Source: CAD feature listing. Evaluate the final solid. Frame: model axes, mm. A direction names the side the tool comes from. Give positions to 0.01 mm unless a question says otherwise; leave off trailing zeros. Loops run counter-clockwise (first coordinate to the right, second up) from the corner with the lowest first, then second, coordinate; pieces in that order, holes last. Notation, with made-up numbers: M -25,-6.5 L 17,-6.5 A34 ccw 17,32.5 Z; hole C 25,76 d10. An arc over 180 degrees is marked long. Put each result on its own line as item: value. Start each with the question number.
```python
from build123d import *

# Parameters (mm, degrees)
F0_R     = 1.539144
F0_R_2   = 1.452362
F0_R_3   = 1.631379
F0_R_4   = 1.528566
F0_R_5   = 1.549722
F0_R_6   = 5.024672
F0_R_7   = 1.528565
F1_DEPTH = 4


with BuildPart() as f1:
    # F0 (on Top) → F1 (new body)
    with BuildSketch(Plane.XY):
        Polygon((18.500502, 18), (-35.499498, 18), (-35.499498, 0), (18.500502, 0), (30.500502, -7), (42.500502, -7), (54.500502, 0), (54.500502, 18), (42.500502, 25), (30.500502, 25), align=None)
        with Locations((-28.499498, 3.5)):
            Circle(F0_R, mode=Mode.SUBTRACT)
        with Locations((29.135042, 3)):
            Circle(F0_R_2, mode=Mode.SUBTRACT)
        with Locations((41.504552, 2.758247)):
            Circle(F0_R_3, mode=Mode.SUBTRACT)
        with Locations((-28.499498, 14.5)):
            Circle(F0_R_4, mode=Mode.SUBTRACT)
        with Locations((31.46798, 15.21882)):
            Circle(F0_R_5, mode=Mode.SUBTRACT)
        with Locations((36.500502, 9)):
            Circle(F0_R_6, mode=Mode.SUBTRACT)
        with Locations((43.865962, 15)):
            Circle(F0_R_7, mode=Mode.SUBTRACT)
    extrude(amount=F1_DEPTH)


solid = f1.part
```
1. Section A-A, the plane y = 9. Output: boundary loops of the cut face in (x, z), plus the area to 3 significant figures.
2. Pull-direction query (X, two-part tool) for faces 4 (the face through (37, 25, 2)), 5 (the face through (54.501, 9, 2)), 6 (the face through (39.875, 2.83, 1.972)); classes: released by +X, released by -X, zero draft, split by the parting line, or undercut.
3. Section C-C, the plane x = 8. Output: boundary loops of the cut face in (y, z), plus the area to 3 significant figures.
4. Section D-D, the plane y = 19.5. Output: boundary loops of the cut face in (x, z).
5. Ray query, line 1 (Y direction, x = 8.5, z = 3.8); line 2 (X direction, y = 5.5, z = 0.3); line 3 (Y direction, x = 34, z = 3.6). Return the intervals inside material, ascending.
6. Set-up query: faces 1 (the face through (-9, 0, 2)), 2 (the face through (36, -7, 2)), 3 (the face through (-8, 18, 2)). Return all of +Z, -Z, +X, -X, +Y, -Y with unobstructed straight access to the full face (end or side cutting, diameter ignored); none if empty.
7. Contact query for flat-ended pins moving along their axis: pin 1 (1.9 mm diameter, centred on x = 31.47, y = 15.22, fed in from -Z); pin 2 (1 mm diameter, centred on x = 44.5, z = 1.5, fed in from -Y); pin 3 (1.2 mm diameter, centred on x = -21, z = 1.5, fed in from -Y). Output: stop coordinate, or through.
8. Section B-B, the plane z = 2.5. Output: boundary loops of the cut face in (x, y).
Results found:
1. outline: M -35.5,0 L 31.48,0 L 31.48,4 L -35.5,4 Z; M 41.53,0 L 54.5,0 L 54.5,4 L 41.53,4 Z
1. area: 320 mm²
2. face 4: zero draft
2. face 5: released by +X
2. face 6: undercut
3. outline: M 0,0 L 18,0 L 18,4 L 0,4 Z
3. area: 72.0 mm²
4. outline: M 21.07,0 L 51.93,0 L 51.93,4 L 21.07,4 Z
5. line 1: 0 to 18
5. line 2: -35.5 to 32.9, 40.11 to 54.5
5. line 3: -7 to 4.64, 13.36 to 25
6. face 1: +Z, -Z, -X, -Y
6. face 2: +Z, -Z, +X, -X, -Y
6. face 3: +Z, -Z, -X, +Y
7. pin 1: through
7. pin 2: y = -6.13
7. pin 3: y = 0
8. outline: M -35.5,0 L 18.5,0 L 30.5,-7 L 42.5,-7 L 54.5,0 L 54.5,18 L 42.5,25 L 30.5,25 L 18.5,18 L -35.5,18 Z; hole C -28.5,3.5 d3.08; hole C -28.5,14.5 d3.06; hole C 29.14,3 d2.9; hole C 31.47,15.22 d3.1; hole C 36.5,9 d10.05; hole C 41.5,2.76 d3.26; hole C 43.87,15 d3.06
